Drawing for the job (mm, zero at the part's lowest x, y, z). Round coordinates to 2 decimals unless told otherwise and drop trailing zeros. Write each loop counter-clockwise with the first axis right and the second up, starting at its lowest first coordinate (ties: lowest second). Pieces come first, ordered by that corner, then holes.
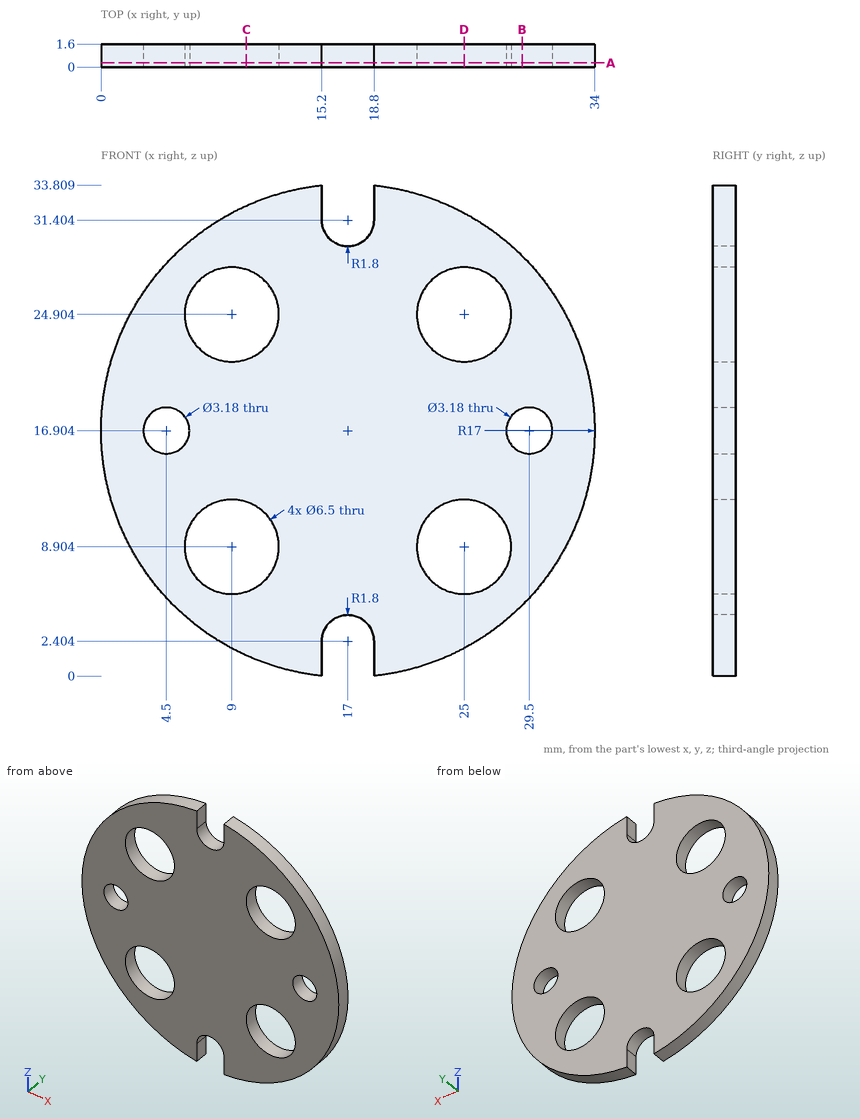
1) Cut at D-D on x = 25. List the corners of the cut face in (y, z) (1 decimal), and give its area (3 significant figures).
2) Flat gauge pin, fed straight in: pin 1 Ø5 at (x, z) = (25, 24.9) entering from +Y. Where does the tip first touch, or does it go through?
3) Wall check: probe 1 along Z at (x, y) = (24, 0.9) (1 decimal); probe 2 along X at (y, z) = (0.6, 25.5) (1 decimal); probe 3 along X at (y, z) = (0.5, 23) (1 decimal). Give the ranges that are in metal, low to high.
4) Cut at C-C on x = 10. List the corners of the cut face in (y, z).
5) Cut at B-B on x = 29. List the corners of the cut face in (y, z) (1 decimal).
6) Cut at A-A on y = 0.3. Give the number of separate pieces and of enclosed holes in the cut face.
Result sheet:
1. outline: (0, 1.9) - (1.6, 1.9) - (1.6, 5.7) - (0, 5.7) - close; (0, 12.2) - (1.6, 12.2) - (1.6, 21.7) - (0, 21.7) - close; (0, 28.2) - (1.6, 28.2) - (1.6, 31.9) - (0, 31.9) - close
1. area: 27.2 mm2
2. pin 1: passes through
3. probe 1: z = 1.4 to 5.8, 12 to 21.8, 28 to 32.4
3. probe 2: x = 2.3 to 5.8, 12.2 to 21.8, 28.2 to 31.7
3. probe 3: x = 1.1 to 6.4, 11.6 to 22.4, 27.6 to 32.9
4. outline: (0, 1.41) - (1.6, 1.41) - (1.6, 5.81) - (0, 5.81) - close; (0, 12) - (1.6, 12) - (1.6, 21.81) - (0, 21.81) - close; (0, 28) - (1.6, 28) - (1.6, 32.4) - (0, 32.4) - close
5. outline: (0, 4.9) - (1.6, 4.9) - (1.6, 15.4) - (0, 15.4) - close; (0, 18.4) - (1.6, 18.4) - (1.6, 28.9) - (0, 28.9) - close
6. separate pieces: 1
6. enclosed holes: 6
